Here's how the part is built. I have some questions about the finished solid (model axes, mm). A direction names the side the tool comes from. Give positions to 0.01 mm unless a question says otherwise; leave off trailing zeros. Write each loop counter-clockwise with the first axis right and the second up, starting at its lowest first coordinate (ties: lowest second). Pieces come first, ordered by that corner, then holes. Notation, with made-up numbers: (-17, 73) -> (5, 73) arc R19 cw to (5, 110) -> close; hole circle Ø6 at (32.5, -39). An arc over 180 degrees is marked (long way). Put each result on its own line as item: value. Start each with the question number.
from build123d import *

# Parameters (mm, degrees)
SKETCH1_W      = 19.05
SKETCH1_H      = 19.05
SKETCH1_R      = 0.889
EXTRUDE1_DEPTH = 2.54
EXTRUDE2_DEPTH = 2.54


with BuildPart() as part:
    # Sketch1 → Extrude1 (new body)
    with BuildSketch(Plane.XY):
        Rectangle(SKETCH1_W, SKETCH1_H)
        Circle(SKETCH1_R, mode=Mode.SUBTRACT)
    extrude(amount=-EXTRUDE1_DEPTH)

    # Sketch2 → Extrude2 (add)
    with BuildSketch(Plane.XY):
        Polygon((0.841446987, 7.7978), (1.397, 1.4478), (-0.8128, 1.4478), (-0.257246987, 7.7978), align=None)
    extrude(amount=EXTRUDE2_DEPTH)


solid = part.part
1) Which directions (+Z, -Z, +X, -X, +Y, -Y) give clear straight access to the entire face, cutting with the end or side of a thin tool? Please do faces 1 (the flat face through (-0.54, 4.58, 1.25)), 2 (the flat face through (0, 1.448, 1)), 3 (the flat face through (1.115, 4.667, 1.252)), 4 (the flat face through (0, 7.798, 1)), 5 (the flat face through (9.525, 0, -1)).
2) I want a section at A-A, the plane x = 0. Write out the boundary of the cut face in (y, z) (3 decimals).
3) I need wall thicknesses on probe 1 along Y at (x, z) = (0, -2) (3 decimals); probe 2 along Z at (x, y) = (3.5, 3.5); probe 3 along X at (y, z) = (6.25, 1.1). Which ranges of each line are inside material? Lowest first, please.
4) I want a section at C-C, the plane y = 7.5. Write out the boundary of the cut face in (x, z) (1 decimal).
5) I want a section at B-B, the plane y = 0. Write out the boundary of the cut face in (x, z) (3 decimals), and give its area (3 significant figures).
6) I'm going to push flat-ended pins straight in: pin 1 Ø1.1 at (x, z) = (0, 1.5) entering from -Y; pin 2 Ø0.5 at (x, z) = (0, 2) entering from +Y; pin 3 Ø1 at (y, z) = (2, 1.5) entering from +X; pin 4 Ø1.1 at (x, y) = (0, 0) entering from +Z. Where does each tip first touch, or does it pass through?
7) Thinking about a two-plate mould opening in Y: for faces 6 (the flat face through (0, -9.525, -1)), 7 (the flat face through (-9.525, 0, -1)), 8 (the cylindrical face through (-0.19, -0.87, -1.25)), which applies, released by +Y, released by -Y, zero draft, split by the parting line, or undercut?
8) I want a section at D-D, the plane z = 1.3. Write out the boundary of the cut face in (x, y).
Established:
1. face 1: +Z, -X, +Y
1. face 2: +Z, +X, -X, -Y
1. face 3: +Z, +X, +Y
1. face 4: +Z, +X, -X, +Y
1. face 5: +Z, -Z, +X, +Y, -Y
2. outline: (-9.525, -2.54) -> (-0.889, -2.54) -> (-0.889, 0) -> (-9.525, 0) -> close; (0.889, -2.54) -> (9.525, -2.54) -> (9.525, 0) -> (7.798, 0) -> (7.798, 2.54) -> (1.448, 2.54) -> (1.448, 0) -> (0.889, 0) -> close
3. probe 1: y = -9.525 to -0.889, 0.889 to 9.525
3. probe 2: z = -2.54 to 0
3. probe 3: x = -0.39 to 0.98
4. outline: (-9.5, -2.5) -> (9.5, -2.5) -> (9.5, 0) -> (0.9, 0) -> (0.9, 2.5) -> (-0.3, 2.5) -> (-0.3, 0) -> (-9.5, 0) -> close
5. outline: (-9.525, -2.54) -> (-0.889, -2.54) -> (-0.889, 0) -> (-9.525, 0) -> close; (0.889, -2.54) -> (9.525, -2.54) -> (9.525, 0) -> (0.889, 0) -> close
5. area: 43.9 mm2
6. pin 1: stops at y = 1.45
6. pin 2: stops at y = 7.8
6. pin 3: stops at x = 1.39
6. pin 4: passes through
7. face 6: released by -Y
7. face 7: zero draft
7. face 8: undercut
8. outline: (-0.81, 1.45) -> (1.4, 1.45) -> (0.84, 7.8) -> (-0.26, 7.8) -> close
